from build123d import *

# Parameters (mm, degrees)
SKETCH1_R           = 16
SKETCH1_R_2         = 7
SKETCH1_R_3         = 2
BOSS_EXTRUDE1_DEPTH = 4.5
CHAMFER1_SIZE       = 1


with BuildPart() as part:
    # Sketch1 → Boss-Extrude1 (new body)
    with BuildSketch(Plane(origin=(0, 0, 0), x_dir=(1, 0, 0), z_dir=(0, 1, 0))):
        Circle(SKETCH1_R)
        Circle(SKETCH1_R_2, mode=Mode.SUBTRACT)
        with Locations((0, 12.5)):
            Circle(SKETCH1_R_3, mode=Mode.SUBTRACT)
        with Locations((12.5, 0)):
            Circle(SKETCH1_R_3, mode=Mode.SUBTRACT)
        with Locations((0, -12.5)):
            Circle(SKETCH1_R_3, mode=Mode.SUBTRACT)
        with Locations((-12.5, 0)):
            Circle(SKETCH1_R_3, mode=Mode.SUBTRACT)
    extrude(amount=BOSS_EXTRUDE1_DEPTH)

    # Chamfer1
    chamfer1_edges = [part.edges().sort_by_distance(p)[0] for p in [
        (10.5, 0, 0),
        (10.5, 4.5, 0),
        (-2, 0, 12.5),
        (-2, 4.5, 12.5),
        (-14.5, 0, 0),
        (-14.5, 4.5, 0),
        (-7, 0, 0),
        (-7, 4.5, 0),
        (-2, 0, -12.5),
        (-2, 4.5, -12.5),
    ]]
    chamfer(chamfer1_edges, length=CHAMFER1_SIZE)


solid = part.part
Could you check a few things on this model? Use its own coordinates, in mm. Round coordinates to 2 decimals unless told otherwise and drop trailing zeros. Loops run counter-clockwise (first coordinate to the right, second up) from the corner with the lowest first, then second, coordinate; pieces in that order, holes last. Notation, with made-up numbers: (38, -23.75) - (90, -23.75) arc R25 ccw to (90, -10.75) - close; hole circle Ø11 at (-27.75, 23.25). An arc over 180 degrees is marked (long way). Write item = value, one per line.
1) If we mould it in two halves opening along X, with no side actions, what happens to faces 1 (the cylindrical face through (-3.47, 2.22, 15.62)), 2 (the flat face through (-7.3, 4.5, -3.8)), 3 (the cylindrical face through (6.466, 2.232, 2.681))? For each: pulls with the +X half, pulls with the -X half, needs draft (parallel to the pull), parting line crosses it, or undercut.
Computed:
face_1 = parting line crosses it
face_2 = needs draft
face_3 = undercut
2) Imagine slicing it at B-B (y = 1.4). Please give me the cut outline in (x, z), and give its area (3 significant figures).
Computed:
outline = circle Ø32 at (0, 0); hole circle Ø4 at (-12.5, 0); hole circle Ø14 at (0, 0); hole circle Ø4 at (0, -12.5); hole circle Ø4 at (0, 12.5); hole circle Ø4 at (12.5, 0)
area = 600 mm2
3) I need wall thicknesses on line 1 along Z through (x, y) = (0, 1.85); line 2 along Z through (x, y) = (-0.5, 2.25). Which ranges of each line are inside material? Lowest first, please. Write a range as from..to.
Computed:
line_1 = -16..-14.5, -10.5..-7, 7..10.5, 14.5..16
line_2 = -15.99..-14.44, -10.56..-6.98, 6.98..10.56, 14.44..15.99
4) Imagine slicing it at A-A (z = 0). Please give me the cut outline in (x, y), and give its area (3 significant figures).
Computed:
outline = (-16, 0) - (-15.5, 0) - (-14.5, 1) - (-14.5, 3.5) - (-15.5, 4.5) - (-16, 4.5) - close; (-10.5, 1) - (-9.5, 0) - (-8, 0) - (-7, 1) - (-7, 3.5) - (-8, 4.5) - (-9.5, 4.5) - (-10.5, 3.5) - close; (7, 1) - (8, 0) - (9.5, 0) - (10.5, 1) - (10.5, 3.5) - (9.5, 4.5) - (8, 4.5) - (7, 3.5) - close; (14.5, 1) - (15.5, 0) - (16, 0) - (16, 4.5) - (15.5, 4.5) - (14.5, 3.5) - close
area = 39.0 mm2
5) Imagine slicing it at D-D (z = 12.5). Please give me the cut outline in (x, y).
Computed:
outline = (-9.99, 0) - (-3, 0) - (-2, 1) - (-2, 3.5) - (-3, 4.5) - (-9.99, 4.5) - close; (2, 1) - (3, 0) - (9.99, 0) - (9.99, 4.5) - (3, 4.5) - (2, 3.5) - close
6) I'm going to push flat-ended pins straight in: P1, Ø2, axis at x = 0.5, z = 9.5, coming from the -Y side; P2, Ø2.5, axis at x = -12.5, z = 0, coming from the -Y side; P3, Ø5, axis at x = 0, z = -12.5, coming from the +Y side; P4, Ø2, axis at x = 4, y = 1, coming from the -Z side. Where does each tip first touch, or does it pass through?
Computed:
P1 = 0
P2 = through
P3 = 4
P4 = -15.72
7) Imagine slicing it at C-C (x = -12.5). Please give me the cut outline in (y, z).
Computed:
outline = (0, -9.99) - (4.5, -9.99) - (4.5, -3) - (3.5, -2) - (1, -2) - (0, -3) - close; (0, 3) - (1, 2) - (3.5, 2) - (4.5, 3) - (4.5, 9.99) - (0, 9.99) - close
